Job drawing, mm, ordinate dimensions from the low corner. One solid piece. A direction names the side the tool comes from. Give positions to 0.01 mm unless a question says otherwise; leave off trailing zeros. Order: outer loops, then holes, each group sorted by start corner. A loop starts at its lowest first (then second) coordinate and runs counter-clockwise, first axis right, second up. Notation, with made-up numbers: M -37,59 L -25,59 A26 ccw -25,86 Z; hole C -1,24 d5. An arc over 180 degrees is marked long. One line per question, with ' | ' between items.
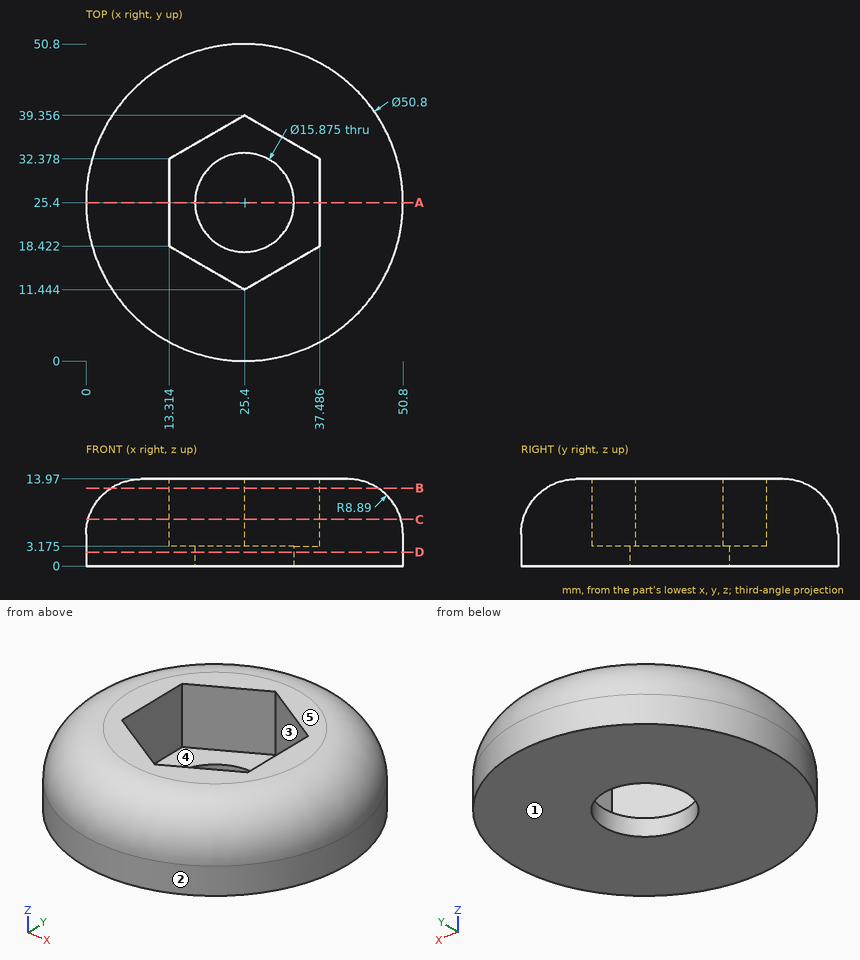
1. Slice it at D-D on z = 2.25. Give the cut face in (x, y) (1 decimal).
Worked out:
outline: C 25.4,25.4 d50.8; hole C 25.4,25.4 d15.9
2. Drop flat-ended pins along their axis: pin 1 (8 mm diameter, centred on x = 12.5, z = 10.5, fed in from -Y); pin 2 (5 mm diameter, centred on x = 38, y = 16.5, fed in from -Z); pin 3 (1.5 mm diameter, centred on x = 30, y = 33.5, fed in from +Z) (3 decimals); pin 4 (1.5 mm diameter, centred on y = 36, z = 6.5, fed in from -X). Give the stop position or say it passes through.
Worked out:
pin 1: stops at y = 2.49 | pin 2: stops at z = 0 | pin 3: stops at z = 3.175 | pin 4: stops at x = 2.09
3. Slice it at C-C on z = 7.5. Give the cut face in (x, y) (1 decimal).
Worked out:
outline: C 25.4,25.4 d50.1; hole M 13.3,18.4 L 25.4,11.4 L 37.5,18.4 L 37.5,32.4 L 25.4,39.4 L 13.3,32.4 Z
4. Slice it at B-B on z = 12.5. Give the cut face in (x, y).
Worked out:
outline: C 25.4,25.4 d42.81; hole M 13.31,18.42 L 25.4,11.44 L 37.49,18.42 L 37.49,32.38 L 25.4,39.36 L 13.31,32.38 Z
5. Slice it at A-A on y = 25.4. Give the cut face in (x, z) (1 decimal).
Worked out:
outline: M 0,0 L 17.5,0 L 17.5,3.2 L 13.3,3.2 L 13.3,14 L 8.9,14 A8.9 ccw 0,5.1 Z; M 33.3,0 L 50.8,0 L 50.8,5.1 A8.9 ccw 41.9,14 L 37.5,14 L 37.5,3.2 L 33.3,3.2 Z
6. Tool access for the marked faces 4 and 5: list every direction of +Z, -Z, +X, -X, +Y, -Y with a clear straight run to the whole face (end or side of a thin tool).
Worked out:
face 4: +Z | face 5: +Z, +X, -X, +Y, -Y
7. Probe L1, parallel to Y at x = 25.4, z = 1.1; L2, parallel to Z at x = 21, y = 35 (1 decimal); L3, parallel to X at y = 27.5, z = 1.5 (1 decimal). List the from-to ranges inside material, lowest first. Write a range as from..to.
Worked out:
L1: y = 0..17.46, 33.34..50.8 | L2: z = 0..3.2 | L3: x = 0.1..17.7, 33.1..50.7
8. Mould opens along Y. For the marked faces 1, 2 and 3 say: released by +Y, released by -Y, zero draft, split by the parting line, or undercut.
Worked out:
face 1: zero draft | face 2: split by the parting line | face 3: undercut
